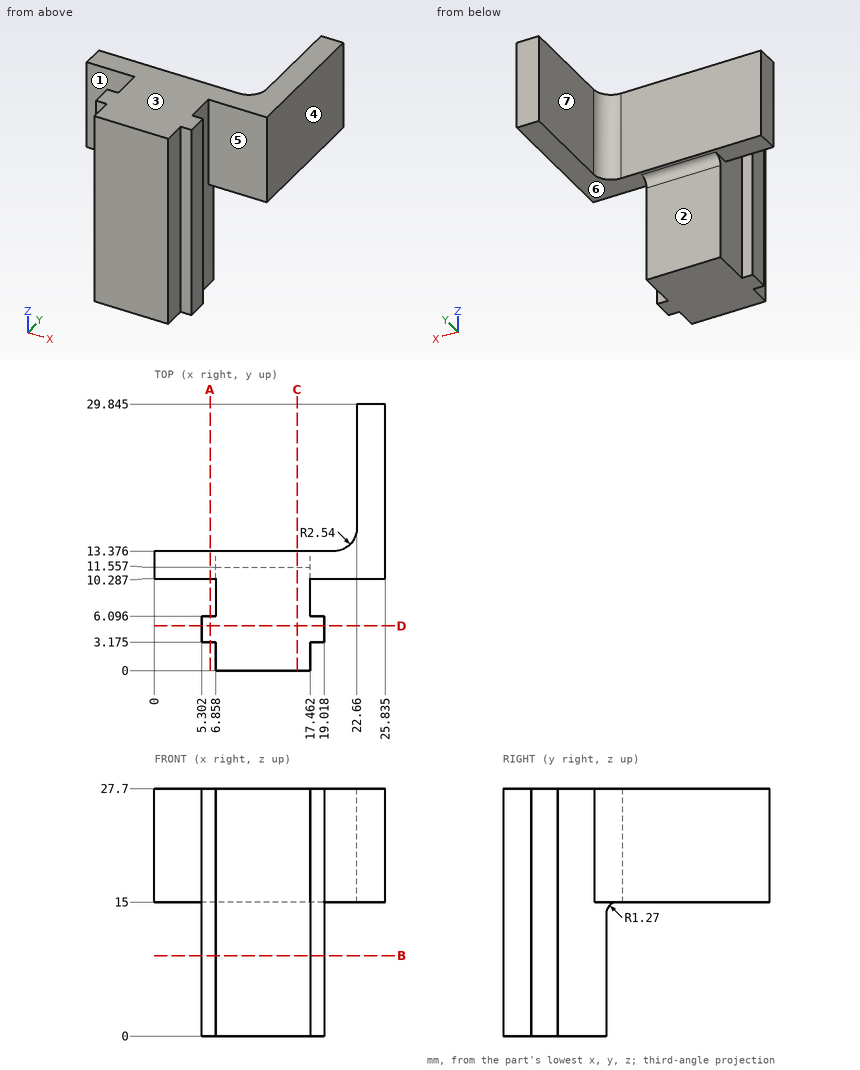
Geometry: see drawing. Coordinates: mm, zero at the bounding-box minimum. A direction names the side the tool comes from. Round coordinates to 2 decimals unless told otherwise and drop trailing zeros. Write each loop counter-clockwise with the first axis right and the second up, starting at its lowest first coordinate (ties: lowest second). Pieces come first, ordered by that corner, then holes. Notation, with made-up numbers: M 55.25,5 L 66.25,5 A21 cw 66.25,13 Z; hole C 74,-20.75 d8. An arc over 180 degrees is marked long. Answer in a Markdown table with one row per item. Add a question column.
(1) Reachability of the marked faces 4, 5, 6 and 7 from +Z, -Z, +X, -X, +Y, -Y: full face, straight path, thin tool, end or side. Return the list, or none.
(2) Cut plane B-B, the plane z = 9. Return the cut outline in (x, y) (1 decimal).
(3) Draft query along Y for the marked faces 1, 2 and 3. Return one class per face: pulls with the +Y half, pulls with the -Y half, needs draft (parallel to the pull), parting line crosses it, or undercut.
(4) Contact query for flat-ended pins moving along their axis: pin 1 (1.5 mm diameter, centred on y = 4.5, z = 15, fed in from -X); pin 2 (0.8 mm diameter, centred on x = 18.5, z = 18, fed in from -Y) (1 decimal); pin 3 (6.5 mm diameter, centred on x = 14.5, z = 19, fed in from +Y). Output: stop coordinate, or through.
(5) Cut plane C-C, the plane x = 16. Return the cut outline in (y, z) (1 decimal).
(6) Ray query, L1, parallel to Y at x = 13.75, z = 20 (1 decimal); L2, parallel to X at y = 28, z = 22 (1 decimal); L3, parallel to Y at x = 8.75, z = 13.25. Return the intervals inside material, ascending.
(7) Cut plane D-D, the plane y = 5. Return the cut outline in (x, z), then the cut area to 3 significant figures.
(8) Cut plane A-A, the plane x = 6.25. Return the cut outline in (y, z) (1 decimal), then the cut area to 3 significant figures.
Established:
| question | item | result |
|---|---|---|
| 1 | face 4 | +Z, -Z, +X, +Y, -Y |
| 1 | face 5 | +Z, -Z, +X |
| 1 | face 6 | -Z, +Y |
| 1 | face 7 | +Z, -Z, -X, +Y |
| 2 | outline | M 5.3,3.2 L 6.9,3.2 L 6.9,0 L 17.5,0 L 17.5,3.2 L 19,3.2 L 19,6.1 L 17.5,6.1 L 17.5,11.6 L 6.9,11.6 L 6.9,6.1 L 5.3,6.1 Z |
| 3 | face 1 | undercut |
| 3 | face 2 | pulls with the +Y half |
| 3 | face 3 | needs draft |
| 4 | pin 1 | x = 5.3 |
| 4 | pin 2 | y = 3.2 |
| 4 | pin 3 | y = 13.38 |
| 5 | outline | M 0,0 L 11.6,0 L 11.6,13.7 A1.3 cw 12.8,15 L 13.4,15 L 13.4,27.7 L 0,27.7 Z |
| 6 | L1 | 0 to 13.4 |
| 6 | L2 | 22.7 to 25.8 |
| 6 | L3 | 0 to 11.56 |
| 7 | outline | M 5.3,0 L 19.02,0 L 19.02,27.7 L 5.3,27.7 Z |
| 7 | area | 380 mm² |
| 8 | outline | M 3.2,0 L 6.1,0 L 6.1,27.7 L 3.2,27.7 Z; M 10.3,15 L 13.4,15 L 13.4,27.7 L 10.3,27.7 Z |
| 8 | area | 120 mm² |
